Part model, mm, in its own coordinate system. A direction names the side the tool comes from. Give positions to 0.01 mm unless a question says otherwise; leave off trailing zeros. Write each loop counter-clockwise with the first axis right and the second up, starting at its lowest first coordinate (ties: lowest second). Pieces come first, ordered by that corner, then holes. Notation, with made-up numbers: M 32.25,-20 L 54.25,-20 A27 ccw 54.25,11 Z; hole C 72.5,45.5 d3. An arc over 180 degrees is marked long. Use CSV: the item, a comma, the result in double quotes. Start each with the question number.
1. Mould opens along X. For faces 5 (the face through (0, -4, 4)), 6 (the face through (18, -2, 4)), 7 (the face through (-8, -2, 4)) say: pulls with the +X half, pulls with the -X half, needs draft (parallel to the pull), parting line crosses it, or undercut.
2. Band-saw the part on B-B, the plane z = 5.5. List the corners of the cut face in (x, y).
3. Band-saw the part on C-C, the plane x = -5. List the corners of the cut face in (y, z).
4. Drop flat-ended pins along their axis: pin 1 Ø3 at (x, z) = (-0.5, 5.5) entering from +Y; pin 2 Ø1.5 at (y, z) = (7, 1.5) entering from -X. Give the stop position or say it passes through.
5. Band-saw the part on A-A, the plane y = 4.5. List the corners of the cut face in (x, z).
6. Band-saw the part on D-D, the plane y = 6.5. List the corners of the cut face in (x, z).
7. Drill centre lines: line 1 along X through (y, z) = (-1.25, 6); line 2 along Y through (x, z) = (31, 5.25); line 3 along X through (y, z) = (1.25, 6). Where is each one in solid material? Low to high. Write a range as from..to.
8. 3-axis set-ups, long thin cutter, end or side, ignore diameter. For faces 1 (the face through (8, -2, 4)), 2 (the face through (13, 9, 4)), 3 (the face through (28, 0, 4)), 4 (the face through (-2, 0, 4)): which of +Z, -Z, +X, -X, +Y, -Y reach the whole face in a straight line?
from build123d import *

# Parameters (mm, degrees)
BOSS_EXTRUDE1_DEPTH = 8


with BuildPart() as part:
    # Sketch2 → Boss-Extrude1 (new body)
    with BuildSketch(Plane.XY):
        with BuildLine():
            Line((0, -4), (8, -4))
            Line((8, -4), (8, 0))
            ThreePointArc((8, 0), (13, 5), (18, 0))
            Line((18, 0), (18, -4))
            Line((18, -4), (34, -4))
            Line((34, -4), (34, 0))
            Line((34, 0), (22, 0))
            ThreePointArc((22, 0), (13, 9), (4, 0))
            Line((4, 0), (-8, 0))
            Line((-8, 0), (-8, -4))
            Line((-8, -4), (0, -4))
        make_face()
    extrude(amount=BOSS_EXTRUDE1_DEPTH)


solid = part.part
Output:
1,face 5,"needs draft"
1,face 6,"undercut"
1,face 7,"pulls with the -X half"
2,outline,"M -8,-4 L 8,-4 L 8,0 A5 cw 18,0 L 18,-4 L 34,-4 L 34,0 L 22,0 A9 ccw 4,0 L -8,0 Z"
3,outline,"M -4,0 L 0,0 L 0,8 L -4,8 Z"
4,pin 1,"stops at y = 0"
4,pin 2,"stops at x = 6.52"
5,outline,"M 5.21,0 L 10.82,0 L 10.82,8 L 5.21,8 Z; M 15.18,0 L 20.79,0 L 20.79,8 L 15.18,8 Z"
6,outline,"M 6.78,0 L 19.22,0 L 19.22,8 L 6.78,8 Z"
7,line 1,"x = -8..8, 18..34"
7,line 2,"y = -4..0"
7,line 3,"x = 4.09..8.16, 17.84..21.91"
8,face 1,"+Z, -Z, -Y"
8,face 2,"+Z, -Z, +Y"
8,face 3,"+Z, -Z, +X, +Y"
8,face 4,"+Z, -Z, -X, +Y"
